For this review, use the dimensioned drawing (mm, ordinates from the lowest corner) and the shaded views. Give positions to 0.01 mm unless a question says otherwise; leave off trailing zeros. Loops run counter-clockwise (first coordinate to the right, second up) from the corner with the lowest first, then second, coordinate; pieces in that order, holes last. Notation, with made-up numbers: (4, -7) - (59, -7) arc R20 cw to (59, 28) - close; hole circle Ø11 at (19, 19). An arc over 180 degrees is marked (long way). Write each question's results on one line, items separated by ' | '.
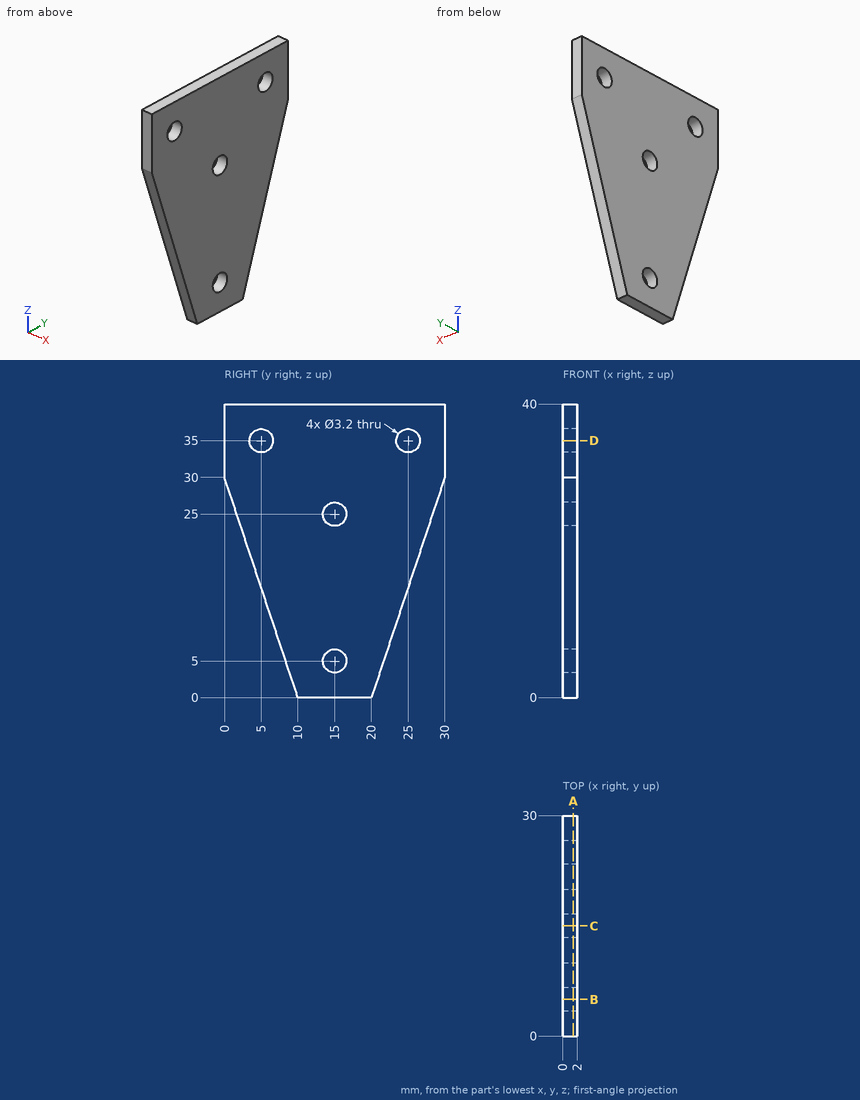
Item 1: We need section B-B on y = 5. Give the boundary of the cut face in (x, z).
Output values:
outline: (0, 15) - (2, 15) - (2, 33.4) - (0, 33.4) - close; (0, 36.6) - (2, 36.6) - (2, 40) - (0, 40) - close
Item 2: We need section C-C on y = 15. Give the boundary of the cut face in (x, z), then the cut area to 3 significant figures.
Output values:
outline: (0, 0) - (2, 0) - (2, 3.4) - (0, 3.4) - close; (0, 6.6) - (2, 6.6) - (2, 23.4) - (0, 23.4) - close; (0, 26.6) - (2, 26.6) - (2, 40) - (0, 40) - close | area: 67.2 mm²
Item 3: Wall thickness on probe 1 along Y at (x, z) = (0.75, 35); probe 2 along Z at (x, y) = (1.4, 14.5); probe 3 along Z at (x, y) = (0.5, 16): over which ranges is each line inside the solid? List them lowest first.
Output values:
probe 1: y = 0 to 3.4, 6.6 to 23.4, 26.6 to 30 | probe 2: z = 0 to 3.48, 6.52 to 23.48, 26.52 to 40 | probe 3: z = 0 to 3.75, 6.25 to 23.75, 26.25 to 40
Item 4: We need section A-A on x = 1.45. Give the boundary of the cut face in (y, z), then the cut area to 3 significant figures.
Output values:
outline: (0, 30) - (10, 0) - (20, 0) - (30, 30) - (30, 40) - (0, 40) - close; hole circle Ø3.2 at (5, 35); hole circle Ø3.2 at (15, 5); hole circle Ø3.2 at (15, 25); hole circle Ø3.2 at (25, 35) | area: 868 mm²
Item 5: We need section D-D on z = 35. Give the boundary of the cut face in (x, y).
Output values:
outline: (0, 0) - (2, 0) - (2, 3.4) - (0, 3.4) - close; (0, 6.6) - (2, 6.6) - (2, 23.4) - (0, 23.4) - close; (0, 26.6) - (2, 26.6) - (2, 30) - (0, 30) - close
